from build123d import *

# Parameters (mm, degrees)
F1_DEPTH = 200
F3_DEPTH = 12.5
F5_DEPTH = 200.001
F7_DEPTH = 12.5
F8_W     = 12.42342
F8_H     = 5.245147
F8_H_2   = 3.165806
F8_H_3   = 8.410953
F9_DEPTH = 12.5


with BuildPart() as f1:
    # F0 (on Front) → F1 (new body)
    with BuildSketch(Plane.XZ):
        Polygon((-10, 30), (0, 0), (10, 30), align=None)
    extrude(amount=F1_DEPTH)

    # F2 (on Right) → F3 (cut, symmetric)
    with BuildSketch(Plane.YZ):
        with BuildLine():
            ThreePointArc((-100, 30), (-47.798467, 22.338442), (0, 0))
            Line((0, 0), (0, 30))
            Line((0, 30), (-100, 30))
        make_face()
        with BuildLine():
            ThreePointArc((-200, 0), (-152.201533, 22.338442), (-100, 30))
            Line((-100, 30), (-200, 30))
            Line((-200, 30), (-200, 0))
        make_face()
    extrude(amount=F3_DEPTH, both=True, mode=Mode.SUBTRACT)

    # F4 (on Front) → F5 (cut, through all)
    with BuildSketch(Plane.XZ):
        Polygon((-7, 30), (0, 8), (7, 30), align=None)
    extrude(amount=F5_DEPTH, mode=Mode.SUBTRACT)

    # F6 (on Right) → F7 (cut, symmetric)
    with BuildSketch(Plane.YZ):
        with BuildLine():
            ThreePointArc((-18.35034, 5), (-100, 25), (-181.64966, 5))
            Line((-181.64966, 5), (-18.35034, 5))
        make_face()
    extrude(amount=F7_DEPTH, both=True, mode=Mode.SUBTRACT)

    # F8 (on Right) → F9 (cut, symmetric)
    with BuildSketch(Plane.YZ):
        with Locations((-6.21171, -2.622573)):
            Rectangle(F8_W, F8_H)
        with Locations((-6.21171, 1.582903)):
            Rectangle(F8_W, F8_H_2)
        with Locations((-193.78829, -1.03967)):
            Rectangle(F8_W, F8_H_3)
    extrude(amount=F9_DEPTH, both=True, mode=Mode.SUBTRACT)


solid = f1.part
The model under review builds one solid part; all positions refer to its coordinate system, in mm. Round coordinates to 2 decimals unless told otherwise and drop trailing zeros. Write each loop counter-clockwise with the first axis right and the second up, starting at its lowest first coordinate (ties: lowest second). Pieces come first, ordered by that corner, then holes. Notation, with made-up numbers: M 24.25,-30 L 54.25,-30 A11 cw 54.25,-16 Z; hole C 77.25,-38.75 d1. An arc over 180 degrees is marked long. Use a Markdown table: item, result. Add a question column.
Q1. We need section A-A, the plane z = 21. State the section outline as (x, y) points, plus the area to 3 significant figures.
Q2. Insertion check: pin 1 (1.7 mm diameter, centred on x = 0, y = -114.5, fed in from +Z); pin 2 (0.6 mm diameter, centred on x = 0.5, z = 1, fed in from -Y); pin 3 (2.5 mm diameter, centred on x = -0.5, z = 1.5, fed in from +Y). Each pin has a flat end and moves straight along its axis. Give the tip position at first contact, or say it passes through.
Q3. We need section C-C, the plane x = 4.75. State the section outline as (y, z) points, plus the area to 3 significant figures.
Q4. We need section D-D, the plane y = -108.5. State the section outline as (x, z) points.
Q5. We need section B-B, the plane y = -48. State the section outline as (x, z) points, plus the area to 3 significant figures.
Q6. The part is to be moulded in two halves that separate along Y. For faces 1 (the face through (-1.32, -99.56, 3.96)), 2 (the face through (-6, -100, 25)), say which applies: pulls with the +Y half, pulls with the -Y half, needs draft (parallel to the pull), parting line crosses it, or undercut.
Q7. To check wall thickness, follow line 1 (X direction, y = -133, z = 22); line 2 (Y direction, x = -2.25, z = 10.5); line 3 (Z direction, x = 7.25, y = -131.5). State the ranges of each line that lie inside material, in increasing order.
Findings below:
| question | item | result |
|---|---|---|
| 1 | outline | M -7,-156.47 L -4.14,-156.47 L -4.14,-137.38 L -7,-137.38 Z; M -7,-62.62 L -4.14,-62.62 L -4.14,-43.53 L -7,-43.53 Z; M 4.14,-156.47 L 7,-156.47 L 7,-137.38 L 4.14,-137.38 Z; M 4.14,-62.62 L 7,-62.62 L 7,-43.53 L 4.14,-43.53 Z |
| 1 | area | 219 mm² |
| 2 | pin 1 | stops at z = 5 |
| 2 | pin 2 | stops at y = -187.58 |
| 2 | pin 3 | stops at y = -12.42 |
| 3 | outline | M -173.99,14.25 L -160.69,14.25 A176.67 cw -126.97,22.93 L -150.19,22.93 A181.67 ccw Z; M -73.03,22.93 A176.67 cw -39.31,14.25 L -26.01,14.25 A181.67 ccw -49.81,22.93 Z |
| 3 | area | 292 mm² |
| 4 | outline | M -9.93,29.8 L -8.27,24.8 L -5.34,24.8 L -6.94,29.8 Z; M -1.67,5 L 0,0 L 1.67,5 Z; M 5.34,24.8 L 8.27,24.8 L 9.93,29.8 L 6.94,29.8 Z |
| 5 | outline | M -7.47,22.4 L -5.72,17.17 L -2.92,17.17 L -4.58,22.4 Z; M -1.67,5 L 0,0 L 1.67,5 Z; M 2.92,17.17 L 5.72,17.17 L 7.47,22.4 L 4.58,22.4 Z |
| 5 | area | 38.1 mm² |
| 6 | face 1 | needs draft |
| 6 | face 2 | undercut |
| 7 | line 1 | x = -7.33 to -4.45, 4.45 to 7.33 |
| 7 | line 2 | y = -181.88 to -170.09, -29.91 to -18.12 |
| 7 | line 3 | z = 22.17 to 27.25 |
